```python
from build123d import *

# Parameters (mm, degrees)
BOSS_EXTRUDE1_DEPTH = 12.7
SKETCH2_R           = 2.675
CUT_EXTRUDE1_DEPTH  = 16.24
SKETCH3_W           = 7.62
SKETCH3_H           = 3.81
CUT_EXTRUDE2_DEPTH  = 97.9700001


with BuildPart() as part:
    # Sketch1 → Boss-Extrude1 (new body)
    with BuildSketch(Plane.XY):
        with BuildLine():
            Line((-48.485, 0), (48.485, 0))
            Line((48.485, 0), (48.485, -15.24))
            ThreePointArc((48.485, -15.24), (0, -10.318710494), (-48.485, -15.24))
            Line((-48.485, -15.24), (-48.485, 0))
        make_face()
    extrude(amount=BOSS_EXTRUDE1_DEPTH)

    # Sketch2 → Cut-Extrude1 (cut, through all)
    with BuildSketch(Plane(origin=(0, 0, 0), x_dir=(1, 0, 0), z_dir=(0, 1, 0))):
        with Locations((-41.485, -6.35)):
            Circle(SKETCH2_R)
        with Locations((41.485, -6.35)):
            Circle(SKETCH2_R)
    extrude(amount=-CUT_EXTRUDE1_DEPTH, mode=Mode.SUBTRACT)

    # Sketch3 → Cut-Extrude2 (cut, through all)
    with BuildSketch(Plane(origin=(48.485, 0, 0), x_dir=(0, 0, -1), z_dir=(1, 0, 0))):
        with Locations((-6.35, -13.335)):
            Rectangle(SKETCH3_W, SKETCH3_H)
    extrude(amount=-CUT_EXTRUDE2_DEPTH, mode=Mode.SUBTRACT)


solid = part.part
```
The listing builds one solid part. Answer for the finished solid, in the listing's coordinates (mm). A direction names the side the tool comes from. Coordinates: 2 decimals unless noted, no trailing zeros. Write each loop counter-clockwise with the first axis right and the second up, starting at its lowest first coordinate (ties: lowest second). Pieces come first, ordered by that corner, then holes. Notation, with made-up numbers: (11, 58.25) - (17, 58.25) arc R26 ccw to (17, 94.25) - close; hole circle Ø8 at (84.25, 46). An arc over 180 degrees is marked (long way). Return JSON: item names as keys, results as strings. Group by question number.
1. A cutting plane is placed at B-B, the plane x = 40. Determine the outline of the cut face in (y, z), plus the area to 3 significant figures.
2. A cutting plane is placed at C-C, the plane y = -6.5. Determine the outline of the cut face in (x, z) (3 decimals).
3. Determine the mould class of faces 1 (the flat face through (-41, -13, 10.16)), 2 (the flat face through (-48.485, -8, 6)), 3 (the flat face through (-41, -13, 2.54)), 4 (the flat face through (1, -6, 0)) for opening direction Z: released by +Z, released by -Z, zero draft, split by the parting line, or undercut.
4. A cutting plane is placed at A-A, the plane z = 6.35. Determine the outline of the cut face in (x, y) (3 decimals), plus the area to 3 significant figures.
5. Given pin 1 (7 mm diameter, centred on x = 41.485, z = 6.35, fed in from -Y); pin 2 (5 mm diameter, centred on x = -41.485, z = 6.35, fed in from +Y); pin 3 (3 mm diameter, centred on x = -17, z = 9, fed in from -Y), each flat-ended and moving along its own axis, determine where each tip first touches the part or whether it passes through.
6. A cutting plane is placed at D-D, the plane x = 24. Determine the outline of the cut face in (y, z).
7. Straight lines are drawn through the part: L1, parallel to X at y = -2.25, z = 6.35 (3 decimals); L2, parallel to Y at x = -30.5, z = 3.5; L3, parallel to X at y = -2.75, z = 7 (3 decimals). For each, find the intervals that lie inside material, in ascending order.
8. Which of the six approach directions +Z, -Z, +X, -X, +Y, -Y give full straight-line access (tool end or side, diameter ignored) to faces 5 (the flat face through (36, -11.43, 6)), 6 (the flat face through (48.485, -8, 6))?
Ans:
{
 "1": {"outline": "(-13.66, 0) - (0, 0) - (0, 4.13) - (-11.43, 4.13) - (-11.43, 2.54) - (-13.66, 2.54) - close; (-13.66, 10.16) - (-11.43, 10.16) - (-11.43, 8.57) - (0, 8.57) - (0, 12.7) - (-13.66, 12.7) - close", "area": "106 mm²"},
 "2": {"outline": "(-48.485, 0) - (48.485, 0) - (48.485, 12.7) - (-48.485, 12.7) - close; hole circle Ø5.35 at (-41.485, 6.35); hole circle Ø5.35 at (41.485, 6.35)"},
 "3": {"face 1": "undercut", "face 2": "zero draft", "face 3": "undercut", "face 4": "released by -Z"},
 "4": {"outline": "(-48.485, -11.43) - (-44.16, -11.43) - (-44.16, 0) - (-48.485, 0) - close; (-38.81, -11.43) - (-23.132, -11.43) arc R241.3 cw to (23.132, -11.43) - (38.81, -11.43) - (38.81, 0) - (-38.81, 0) - close; (44.16, -11.43) - (48.485, -11.43) - (48.485, 0) - (44.16, 0) - close", "area": "952 mm²"},
 "5": {"pin 1": "y = -11.43", "pin 2": "through", "pin 3": "y = -11.03"},
 "6": {"outline": "(-11.52, 0) - (0, 0) - (0, 12.7) - (-11.52, 12.7) - (-11.52, 10.16) - (-11.43, 10.16) - (-11.43, 2.54) - (-11.52, 2.54) - close"},
 "7": {"L1": "-48.485 to -44.16, -38.81 to 38.81, 44.16 to 48.485", "L2": "-11.43 to 0", "L3": "-48.485 to -44.08, -38.89 to 38.89, 44.08 to 48.485"},
 "8": {"face 5": "+X, -X, -Y", "face 6": "+Z, -Z, +X, +Y, -Y"}
}
